Solid Edge part; units mm, degrees
sketch "Sketch1" plane through (0, 0, 0) normal (0, -1, 0) x (1, 0, 0)
  line L0 (0, 0) -> (16, 0)
  line L1 (16, 0) -> (16, 4)
  line L2 (16, 4) -> (24.4083, 4)
  line L3 (24.4083, 4) -> (24.4083, 11)
  line L4 (24.4083, 11) -> (38, 11)
  line L5 (38, 11) -> (38, 15)
  arc A0 (0, 23.8599) -> (38, 15) centre (0, -62.0605) cw
  dimension "D1" = 16
  dimension "D2" = 24.4083
revolve "RevolvedProtrusion1" add sketch "Sketch1" angle 360 about axis through (0, 0, 0) along (0, 0, 1)
hole "Hole_1" at (32, 0, 20) direction (0, 0, -1) diameter 5.3 end up to next counterbore diameter 9 counterbore depth 7.8
pattern_circular "Pattern1" count 6 over 360 about axis through (0, 0, 0) along (0, 0, -1) of "Hole_1"
properties material "Bronze, 90%"
Build history of the part. All positions in model axes, mm. A direction names the side the tool comes from. Round coordinates to 2 decimals unless told otherwise and drop trailing zeros. Write each loop counter-clockwise with the first axis right and the second up, starting at its lowest first coordinate (ties: lowest second). Pieces come first, ordered by that corner, then holes.
1) Drill centre lines: probe 1 along Y at (x, z) = (15.5, 16); probe 2 along Y at (x, z) = (16, 15.75); probe 3 along Y at (x, z) = (32, 11.65). Where is each one in solid material? Low to high.
2) Band-saw the part on D-D, the plane z = 9.25. List the corners of the cut face in (x, y), and give its area (3 significant figures).
3) Band-saw the part on A-A, the plane y = 0. List the corners of the cut face in (x, z).
4) Mould opens along Y. For faces 1 (the flat face through (19, 28, 12.2)), 2 (the cylindrical face through (-5.29, -23.83, 7.55)), 3 (the flat face through (16, -5, 4)), 4 (the cylindrical face through (-13.766, -29.137, 11.608)) say: +Y half, -Y half, draft (parallel to the pull), parting line (faces both ways), or undercut.
5) 3-axis set-ups, long thin cutter, end or side, ignore diameter. For faces 5 (the cylindrical face through (-3.47, -15.62, 2.03)), 6 (the cylindrical face through (-34.63, -0.34, 11.61)), 7 (the cylindrical face through (27.54, 0.59, 14.93)): which of +Z, -Z, +X, -X, +Y, -Y reach the whole face in a straight line?
6) Pin check, flat tips, straight feed: pin 1 (4.5 mm diameter, centred on x = 31, y = -0.5, fed in from +Z); pin 2 (8 mm diameter, centred on x = -16, y = -27.71, fed in from -Z); pin 3 (7 mm diameter, centred on x = 14.5, y = -27, fed in from +Z); pin 4 (8 mm diameter, centred on x = 17, y = -5.5, fed in from -Z). Stop position of each tip, or through.
7) Band-saw the part on B-B, the plane x = -32. List the corners of the cut face in (y, z), and give its area (3 significant figures).
8) Band-saw the part on C-C, the plane x = 0. List the corners of the cut face in (y, z).
Ans:
1. probe 1: y = -32.38 to -32.18, -23.24 to 23.24, 32.18 to 32.38
1. probe 2: y = -32.74 to -32.21, -23.21 to 23.21, 32.21 to 32.74
1. probe 3: y = -20.49 to -2.65, 2.65 to 20.49
2. outline: circle Ø48.82 at (0, 0)
2. area: 1,870 mm2
3. outline: (-38, 11) - (-34.65, 11) - (-34.65, 12.2) - (-36.5, 12.2) - (-36.5, 15.72) arc R85.92 ccw to (-38, 15) - close; (-29.35, 11) - (-24.41, 11) - (-24.41, 4) - (-16, 4) - (-16, 0) - (16, 0) - (16, 4) - (24.41, 4) - (24.41, 11) - (29.35, 11) - (29.35, 12.2) - (27.5, 12.2) - (27.5, 19.34) arc R85.92 ccw to (-27.5, 19.34) - (-27.5, 12.2) - (-29.35, 12.2) - close; (34.65, 11) - (38, 11) - (38, 15) arc R85.92 ccw to (36.5, 15.72) - (36.5, 12.2) - (34.65, 12.2) - close
4. face 1: undercut
4. face 2: parting line
4. face 3: draft
4. face 4: undercut
5. face 5: -Z
5. face 6: +Z, -Z
5. face 7: +Z
6. pin 1: stops at z = 12.2
6. pin 2: stops at z = 11
6. pin 3: stops at z = 19.46
6. pin 4: stops at z = 0
7. outline: (-20.49, 11) - (-2.65, 11) - (-2.65, 12.2) - (-4.5, 12.2) - (-4.5, 17.55) arc R79.74 ccw to (-20.49, 15) - close; (2.65, 11) - (20.49, 11) - (20.49, 15) arc R79.74 ccw to (4.5, 17.55) - (4.5, 12.2) - (2.65, 12.2) - close
7. area: 182 mm2
8. outline: (-38, 11) - (-24.41, 11) - (-24.41, 4) - (-16, 4) - (-16, 0) - (16, 0) - (16, 4) - (24.41, 4) - (24.41, 11) - (38, 11) - (38, 15) arc R85.92 ccw to (-38, 15) - close
